Geometry: see drawing. Coordinates: mm, zero at the bounding-box minimum. A direction names the side the tool comes from. Round coordinates to 2 decimals unless told otherwise and drop trailing zeros. Loops run counter-clockwise (first coordinate to the right, second up) from the corner with the lowest first, then second, coordinate; pieces in that order, holes last. Notation, with made-up numbers: M -37,83.25 L -16,83.25 A28 ccw -16,101.25 Z; hole C -7.5,-36 d4. An arc over 180 degrees is marked long. Answer as a JSON object with one key per item and string values.
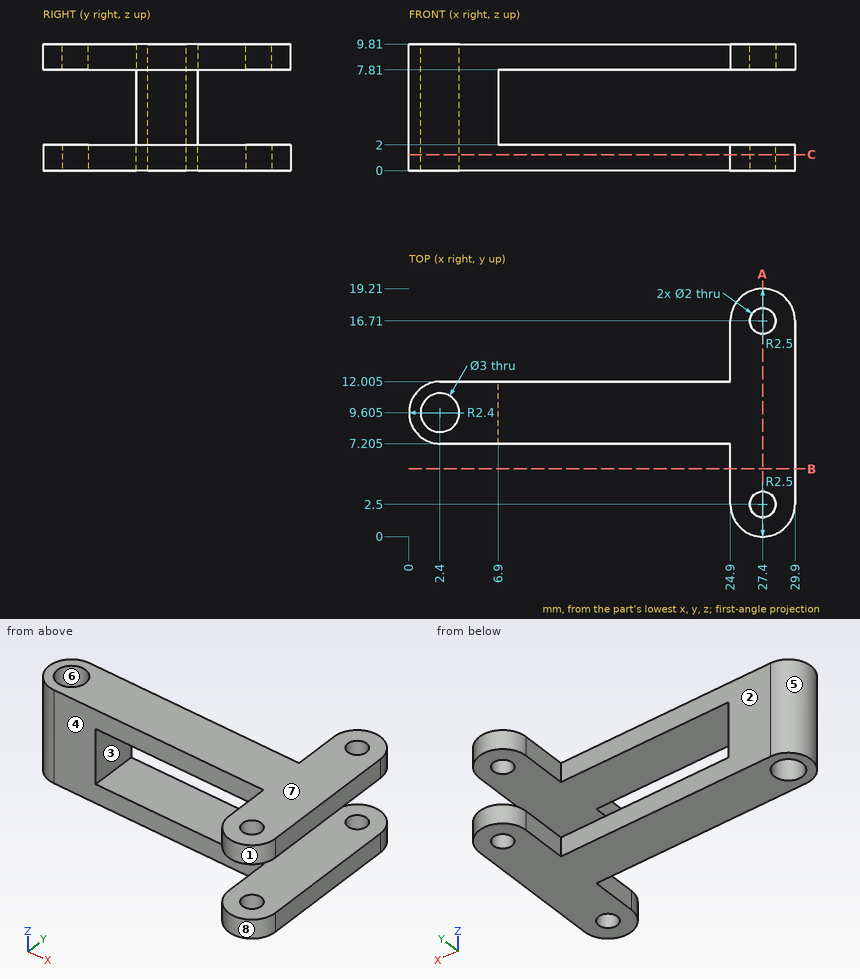
1) Reachability of the marked faces 1, 2, 3 and 4 from +Z, -Z, +X, -X, +Y, -Y: full face, straight path, thin tool, end or side. Return the list, or none.
Results:
{"face 1": "+Z, -Z, -Y", "face 2": "+Z, -Z, -X, +Y", "face 3": "+X, +Y, -Y", "face 4": "+Z, -Z, -X, -Y"}
2) Pin query (flat end, axial travel): P1, Ø1.6, axis at y = 4, z = 9, coming from the -X side; P2, Ø1.5, axis at x = 24, z = 1.5, coming from the +Y side (3 decimals); P3, Ø5, axis at x = 23.5, z = 3.5, coming from the -Y side. Return the tip coordinate at first contact, or that it passes through.
Results:
{"P1": "x = 24.9", "P2": "y = 12.005", "P3": "y = 0.88"}
3) Ray query, line 1 (Y direction, x = 27.4, z = 9.25); line 2 (X direction, y = 2.5, z = 0.65); line 3 (Y direction, x = 2.4, z = 5) (3 decimals). Return the intervals inside material, ascending.
Results:
{"line 1": "0 to 1.5, 3.5 to 15.71, 17.71 to 19.21", "line 2": "24.9 to 26.4, 28.4 to 29.9", "line 3": "7.205 to 8.105, 11.105 to 12.005"}
4) Section query B-B (y = 5.25). Return the cut outline in (x, z), and give its area (3 significant figures).
Results:
{"outline": "M 24.9,0 L 29.9,0 L 29.9,2 L 24.9,2 Z; M 24.9,7.81 L 29.9,7.81 L 29.9,9.81 L 24.9,9.81 Z", "area": "20.0 mm2"}
5) Section query A-A (x = 27.4). Return the cut outline in (y, z).
Results:
{"outline": "M 0,0 L 1.5,0 L 1.5,2 L 0,2 Z; M 0,7.81 L 1.5,7.81 L 1.5,9.81 L 0,9.81 Z; M 3.5,0 L 15.71,0 L 15.71,2 L 3.5,2 Z; M 3.5,7.81 L 15.71,7.81 L 15.71,9.81 L 3.5,9.81 Z; M 17.71,0 L 19.21,0 L 19.21,2 L 17.71,2 Z; M 17.71,7.81 L 19.21,7.81 L 19.21,9.81 L 17.71,9.81 Z"}
6) Pull-direction query (Y, two-part tool) for the marked faces 5, 6, 7 and 8; classes: +Y half, -Y half, draft (parallel to the pull), parting line (faces both ways), or undercut.
Results:
{"face 5": "parting line", "face 6": "undercut", "face 7": "draft", "face 8": "-Y half"}
7) Section query C-C (z = 1.25). Return the cut outline in (x, y) (3 decimals), and give its area (3 significant figures).
Results:
{"outline": "M 2.4,7.205 L 24.9,7.205 L 24.9,2.5 A2.5 ccw 29.9,2.5 L 29.9,16.71 A2.5 ccw 24.9,16.71 L 24.9,12.005 L 2.4,12.005 A2.4 ccw Z; hole C 2.4,9.605 d3; hole C 27.4,2.5 d2; hole C 27.4,16.71 d2", "area": "194 mm2"}
